Can you work these out from the model? Positions are in its coordinate system, mm. Face numbers are marked on the shaded views. A direction names the side the tool comes from. Round coordinates to 2 decimals unless told otherwise and drop trailing zeros. Loops run counter-clockwise (first coordinate to the right, second up) from the corner with the lowest first, then second, coordinate; pieces in that order, holes last. Notation, with made-up numbers: (54, 56) -> (85, 56) arc R16 ccw to (85, 86) -> close; hole circle Ø9 at (57, -7.75). An arc over 180 degrees is marked (long way). Use a Markdown table: item, result.
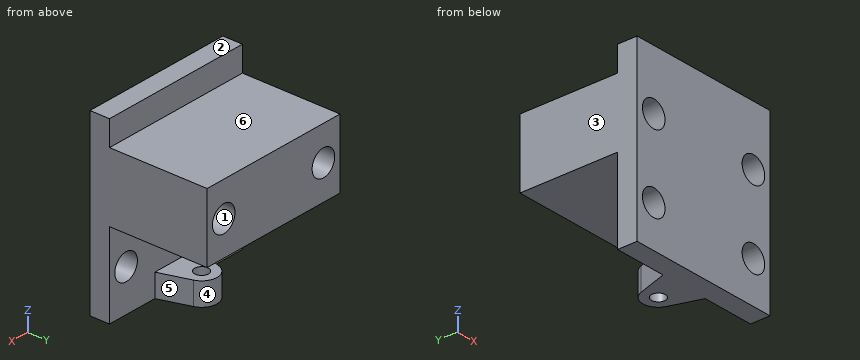
from build123d import *

# Parameters (mm, degrees)
SKETCH036_W  = 19.99996
SKETCH036_H  = 23.09876
SKETCH036_R  = 1.7
PAD003_DEPTH = 2.54
SKETCH051_W  = 19.99996
SKETCH051_H  = 8.89
SKETCH051_R  = 1.7
PAD011_DEPTH = 12.7
SKETCH050_R  = 0.9
PAD012_DEPTH = 2.975


with BuildPart() as part:
    # Sketch036 → Pad003 (new body)
    with BuildSketch(Plane(origin=(0, 10, -45.999574), x_dir=(-1, 0, 0), z_dir=(0, 1, 0))):
        with Locations((0, 1.15062)):
            Rectangle(SKETCH036_W, SKETCH036_H)
        with Locations((-7.5, 5.00124)):
            Circle(SKETCH036_R, mode=Mode.SUBTRACT)
        with Locations((-7.5, -4.99876)):
            Circle(SKETCH036_R, mode=Mode.SUBTRACT)
        with Locations((7.5, -4.99876)):
            Circle(SKETCH036_R, mode=Mode.SUBTRACT)
        with Locations((7.5, 5.00124)):
            Circle(SKETCH036_R, mode=Mode.SUBTRACT)
    extrude(amount=PAD003_DEPTH)

    # Sketch051 (on Face10 of Pad003) → Pad011 (join)
    with BuildSketch(Plane(origin=(0, 12.54, -45.999574), x_dir=(-1, 0, 0), z_dir=(0, 1, 0))):
        with Locations((0, 5.00124)):
            Rectangle(SKETCH051_W, SKETCH051_H)
        with Locations((-7.5, 5.00124)):
            Circle(SKETCH051_R, mode=Mode.SUBTRACT)
        with Locations((7.5, 5.00124)):
            Circle(SKETCH051_R, mode=Mode.SUBTRACT)
    extrude(amount=PAD011_DEPTH)

    # Sketch050 → Pad012 (join)
    with BuildSketch(Plane(origin=(0, 10, -56.398334), x_dir=(-1, 0, 0), z_dir=(0, 0, -1))):
        with BuildLine():
            Line((-3.175, 2.54), (-3.175, 0))
            Line((-3.175, 0), (3.175, 0))
            Line((3.175, 0), (3.175, 2.54))
            Line((3.175, 2.54), (1.90374, 6.488023))
            ThreePointArc((1.90374, 6.488023), (0, 7.87502), (-1.90374, 6.488023))
            Line((-1.90374, 6.488023), (-3.175, 2.54))
        make_face()
        with Locations((0, 5.87502)):
            Circle(SKETCH050_R, mode=Mode.SUBTRACT)
    extrude(amount=-PAD012_DEPTH)


solid = part.part
1. I want a section at D-D (x = 5). Please give me the cut outline in (y, z), plus the area to 3 significant figures.
Answer sheet:
| item | result |
|---|---|
| outline | (10, -56.4) -> (12.54, -56.4) -> (12.54, -45.44) -> (25.24, -45.44) -> (25.24, -36.55) -> (12.54, -36.55) -> (12.54, -33.3) -> (10, -33.3) -> close |
| area | 172 mm² |
2. I want a section at A-A (y = 15.5). Please give me the cut outline in (x, z), plus the area to 3 significant figures.
Answer sheet:
| item | result |
|---|---|
| outline | (-10, -45.44) -> (10, -45.44) -> (10, -36.55) -> (-10, -36.55) -> close; (-2.22, -56.4) -> (-0.82, -56.4) -> (-0.82, -53.42) -> (-2.22, -53.42) -> close; (0.82, -56.4) -> (2.22, -56.4) -> (2.22, -53.42) -> (0.82, -53.42) -> close; hole circle Ø3.4 at (-7.5, -41); hole circle Ø3.4 at (7.5, -41) |
| area | 168 mm² |
3. Will these pins go through, and if not, where does the flat tip stop? pin 1 Ø6.5 at (x, y) = (-3, 21.5) entering from +Z; pin 2 Ø4 at (x, y) = (-5, 17.5) entering from -Z.
Answer sheet:
| item | result |
|---|---|
| pin 1 | stops at z = -36.55 |
| pin 2 | stops at z = -45.44 |
4. Which directions (+Z, -Z, +X, -X, +Y, -Y) give clear straight access to the entire face, cutting with the end or side of a thin tool? Please do the marked faces 4, 5 and 6.
Answer sheet:
| item | result |
|---|---|
| face 4 | -Z, +Y |
| face 5 | -Z, +X, +Y |
| face 6 | +Z, +X, -X, +Y |
5. If we mould it in two halves opening along X, with no side actions, what happens to the marked faces 1, 2 and 3? For each: +X half, -X half, draft (parallel to the pull), parting line (faces both ways), or undercut.
Answer sheet:
| item | result |
|---|---|
| face 1 | undercut |
| face 2 | draft |
| face 3 | -X half |
6. I need wall thicknesses on line 1 (Z direction, x = 7.5, y = 10.7); line 2 (X direction, y = 11.25, z = -52.5); line 3 (Y direction, x = -4.5, z = -50.25). Which ranges of each line are inside material? Lowest first, please.
Answer sheet:
| item | result |
|---|---|
| line 1 | z = -56.4 to -52.7, -49.3 to -42.7, -39.3 to -33.3 |
| line 2 | x = -10 to -8.3, -6.7 to 6.7, 8.3 to 10 |
| line 3 | y = 10 to 12.54 |
7. I want a section at B-B (x = 0). Please give me the cut outline in (y, z), plus the area to 3 significant figures.
Answer sheet:
| item | result |
|---|---|
| outline | (10, -56.4) -> (14.98, -56.4) -> (14.98, -53.42) -> (12.54, -53.42) -> (12.54, -45.44) -> (25.24, -45.44) -> (25.24, -36.55) -> (12.54, -36.55) -> (12.54, -33.3) -> (10, -33.3) -> close; (16.78, -56.4) -> (17.88, -56.4) -> (17.88, -53.42) -> (16.78, -53.42) -> close |
| area | 182 mm² |
8. I want a section at C-C (x = -7.5). Please give me the cut outline in (y, z), plus the area to 3 significant figures.
Answer sheet:
| item | result |
|---|---|
| outline | (10, -56.4) -> (12.54, -56.4) -> (12.54, -52.7) -> (10, -52.7) -> close; (10, -49.3) -> (12.54, -49.3) -> (12.54, -45.44) -> (25.24, -45.44) -> (25.24, -42.7) -> (10, -42.7) -> close; (10, -39.3) -> (25.24, -39.3) -> (25.24, -36.55) -> (12.54, -36.55) -> (12.54, -33.3) -> (10, -33.3) -> close |
| area | 111 mm² |
